from build123d import *

# Parameters (mm, degrees)
F1_DEPTH = 31.75
F2_R     = 1.8288
F3_DEPTH = 5.020116


with BuildPart() as f1:
    # F0 (on Top) → F1 (new body)
    with BuildSketch(Plane.XY):
        with BuildLine():
            ThreePointArc((-18.25625, 3.272715), (-10.222452, 6.942477), (-4.7625, 0))
            Line((-4.7625, 0), (4.7625, 0))
            ThreePointArc((4.7625, 0), (10.222452, 6.942477), (18.25625, 3.272715))
            Line((18.25625, 3.272715), (21.43125, 3.272715))
            ThreePointArc((21.43125, 3.272715), (26.680106, 7.058374), (32.832644, 5.051394))
            Line((32.832644, 5.051394), (33.955176, 6.173926))
            ThreePointArc((33.955176, 6.173926), (26.931061, 8.689759), (20.527766, 4.860215))
            Line((20.527766, 4.860215), (19.159734, 4.860215))
            ThreePointArc((19.159734, 4.860215), (12.003216, 8.730712), (4.7625, 5.020116))
            Line((4.7625, 5.020116), (-4.7625, 5.020116))
            ThreePointArc((-4.7625, 5.020116), (-12.003216, 8.730712), (-19.159734, 4.860215))
            Line((-19.159734, 4.860215), (-20.527766, 4.860215))
            ThreePointArc((-20.527766, 4.860215), (-26.931061, 8.689759), (-33.955176, 6.173926))
            Line((-33.955176, 6.173926), (-32.832644, 5.051394))
            ThreePointArc((-32.832644, 5.051394), (-26.680106, 7.058374), (-21.43125, 3.272715))
            Line((-21.43125, 3.272715), (-18.25625, 3.272715))
        make_face()
    extrude(amount=F1_DEPTH)

    # F2 (on face) → F3 (cut, through all)
    with BuildSketch(Plane(origin=(0, 5.020116, 0), x_dir=(-1, 0, 0), z_dir=(0, 1, 0))):
        with Locations((0, 3.96875)):
            Circle(F2_R)
        with Locations((0, 27.78125)):
            Circle(F2_R)
    extrude(amount=-F3_DEPTH, mode=Mode.SUBTRACT)


solid = f1.part
The model under review builds one solid part; all positions refer to its coordinate system, in mm. A direction names the side the tool comes from. Round coordinates to 2 decimals unless told otherwise and drop trailing zeros. Loops run counter-clockwise (first coordinate to the right, second up) from the corner with the lowest first, then second, coordinate; pieces in that order, holes last. Notation, with made-up numbers: (-12, 83.5) -> (4, 83.5) arc R28 ccw to (4, 113.5) -> close; hole circle Ø3 at (72, 61.25). An arc over 180 degrees is marked (long way). Answer as CSV lines item,"result".
1) Draft analysis for pull direction Z (two halves, no side actions). For faces 1 (the face through (0, 4, 31.75)), 2 (the face through (0.24, 2.55, 5.78)), 3 (the face through (0.396, 2.545, 25.996)), 4 (the face through (-20, 3.273, 16)), state which applies: pulls with the +Z half, pulls with the -Z half, needs draft (parallel to the pull), parting line crosses it, or undercut.
Geometry results:
face 1,"pulls with the +Z half"
face 2,"undercut"
face 3,"undercut"
face 4,"needs draft"
2) Tool access review of faces 5 (the face through (20, 3.273, 16)), 6 (the face through (-20, 4.86, 16)), 7 (the face through (-10.352, 6.973, 15.653)): name each direction out of +Z, -Z, +X, -X, +Y, -Y from which nothing blocks a thin tool from reaching the whole face with its end or side.
Geometry results:
face 5,"+Z, -Z, +X, -Y"
face 6,"+Z, -Z, +Y"
face 7,"+Z, -Z, -Y"
3) Add section C-C on y = 7.75. Write out the cut boundary in (x, z), plus the area to 3 significant figures.
Geometry results:
outline,"(-31.8, 0) -> (-23.76, 0) -> (-23.76, 31.75) -> (-31.8, 31.75) -> close; (-15.93, 0) -> (-7.88, 0) -> (-7.88, 31.75) -> (-15.93, 31.75) -> close; (7.88, 0) -> (15.93, 0) -> (15.93, 31.75) -> (7.88, 31.75) -> close; (23.76, 0) -> (31.8, 0) -> (31.8, 31.75) -> (23.76, 31.75) -> close"
area,"1,020 mm²"
4) For P1, Ø3, axis at x = 11, y = 4, coming from the -Z side; P2, Ø5, axis at y = 1, z = 22.5, coming from the +X side; P3, Ø3.5, axis at x = -19.5, z = 10.5, coming from the -Y side; P4, Ø1, axis at x = 22.5, z = 22.5, coming from the +Y side, all flat-tipped, find the tip position at first contact; note any pin that passes through.
Geometry results:
P1,"passes through"
P2,"stops at x = 21.55"
P3,"stops at y = 3.27"
P4,"stops at y = 7.31"
5) Add section A-A on x = 0. Write out the cut boundary in (y, z), plus the area to 3 significant figures.
Geometry results:
outline,"(0, 0) -> (5.02, 0) -> (5.02, 2.14) -> (0, 2.14) -> close; (0, 5.8) -> (5.02, 5.8) -> (5.02, 25.95) -> (0, 25.95) -> close; (0, 29.61) -> (5.02, 29.61) -> (5.02, 31.75) -> (0, 31.75) -> close"
area,"123 mm²"
6) To check wall thickness, follow line 1 along Z through (x, y) = (0, 2.5); line 2 along X through (y, z) = (7.5, 28); line 3 along X through (y, z) = (4, 11). State the ranges of each line that lie inside material, in increasing order. Write a range as from..to.
Geometry results:
line 1,"z = 0..2.14, 5.8..25.95, 29.61..31.75"
line 2,"x = -32.25..-23.31, -16.38..-7.44, 7.44..16.38, 23.31..32.25"
line 3,"x = -21.86..-17.83, -5.99..5.99, 17.83..21.86"
7) Add section B-B on z = 3. Write out the cut boundary in (x, y).
Geometry results:
outline,"(-33.96, 6.17) -> (-32.83, 5.05) arc R7.14 cw to (-21.43, 3.27) -> (-18.26, 3.27) arc R7.14 cw to (-4.76, 0) -> (-1.55, 0) -> (-1.55, 5.02) -> (-4.76, 5.02) arc R8.73 ccw to (-19.16, 4.86) -> (-20.53, 4.86) arc R8.73 ccw to start; (1.55, 0) -> (4.76, 0) arc R7.14 cw to (18.26, 3.27) -> (21.43, 3.27) arc R7.14 cw to (32.83, 5.05) -> (33.96, 6.17) arc R8.73 ccw to (20.53, 4.86) -> (19.16, 4.86) arc R8.73 ccw to (4.76, 5.02) -> (1.55, 5.02) -> close"
8) Add section D-D on z = 23.5. Write out the cut boundary in (x, y), plus the area to 3 significant figures.
Geometry results:
outline,"(-33.96, 6.17) -> (-32.83, 5.05) arc R7.14 cw to (-21.43, 3.27) -> (-18.26, 3.27) arc R7.14 cw to (-4.76, 0) -> (4.76, 0) arc R7.14 cw to (18.26, 3.27) -> (21.43, 3.27) arc R7.14 cw to (32.83, 5.05) -> (33.96, 6.17) arc R8.73 ccw to (20.53, 4.86) -> (19.16, 4.86) arc R8.73 ccw to (4.76, 5.02) -> (-4.76, 5.02) arc R8.73 ccw to (-19.16, 4.86) -> (-20.53, 4.86) arc R8.73 ccw to start"
area,"156 mm²"
